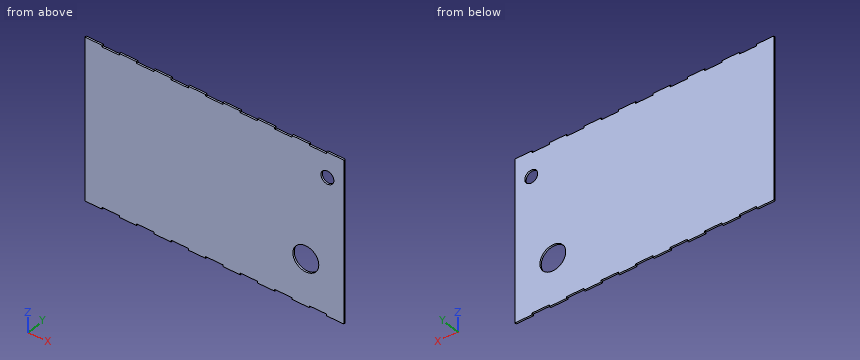
```python
from build123d import *

# Parameters (mm, degrees)
SKETCH1_W               = 300
SKETCH1_H               = 188
BOSS_EXTRUDE1_DEPTH     = 2
SKETCH2_W               = 20
SKETCH2_H               = 2
CUT_EXTRUDE1_DEPTH      = 4
LPATTERN1_COUNT         = 8
LPATTERN1_PITCH         = 40
MIRROR1_COPY_1_SKETCH_W = 20
MIRROR1_COPY_1_SKETCH_H = 2
MIRROR1_COPY_1_DEPTH    = 4
MIRROR1_COPY_2_SKETCH_W = 20
MIRROR1_COPY_2_SKETCH_H = 2
MIRROR1_COPY_2_DEPTH    = 4
MIRROR1_COPY_3_SKETCH_W = 20
MIRROR1_COPY_3_SKETCH_H = 2
MIRROR1_COPY_3_DEPTH    = 4
MIRROR1_COPY_4_SKETCH_W = 20
MIRROR1_COPY_4_SKETCH_H = 2
MIRROR1_COPY_4_DEPTH    = 4
MIRROR1_COPY_5_SKETCH_W = 20
MIRROR1_COPY_5_SKETCH_H = 2
MIRROR1_COPY_5_DEPTH    = 4
MIRROR1_COPY_6_SKETCH_W = 20
MIRROR1_COPY_6_SKETCH_H = 2
MIRROR1_COPY_6_DEPTH    = 4
MIRROR1_COPY_7_SKETCH_W = 20
MIRROR1_COPY_7_SKETCH_H = 2
MIRROR1_COPY_7_DEPTH    = 4
SKETCH4_R               = 7.5
SKETCH4_R_2             = 15
CUT_EXTRUDE2_DEPTH      = 3


with BuildPart() as part:
    # Sketch1 → Boss-Extrude1 (new body)
    with BuildSketch(Plane(origin=(0, 0, 0), x_dir=(1, 0, 0), z_dir=(0, 1, 0))):
        with Locations((-74.28137931, -28.264827586)):
            Rectangle(SKETCH1_W, SKETCH1_H)
    extrude(amount=BOSS_EXTRUDE1_DEPTH)

    # Sketch2 → Cut-Extrude1 (cut)
    with BuildSketch(Plane(origin=(0, 2, 0), x_dir=(1, 0, 0), z_dir=(0, 1, 0))):
        with Locations((-194.28137931, -121.264827586)):
            Rectangle(SKETCH2_W, SKETCH2_H)
    cut_extrude1 = extrude(amount=-CUT_EXTRUDE1_DEPTH, mode=Mode.SUBTRACT)

    # LPattern1: Cut-Extrude1 ×8
    with Locations(*[(i * LPATTERN1_PITCH, 0, 0) for i in range(1, LPATTERN1_COUNT)]):
        add(cut_extrude1, mode=Mode.SUBTRACT)

    # Mirror1: Cut-Extrude1 across plane
    add(cut_extrude1.mirror(Plane.XY.offset(28.264827586)), mode=Mode.SUBTRACT)

    # Mirror1 copy 1 sketch → Mirror1 copy 1 (cut)
    with BuildSketch(Plane(origin=(40, 2, 56.529655172), x_dir=(1, 0, 0), z_dir=(0, 1, 0))):
        with Locations((-194.28137931, 121.264827586)):
            Rectangle(MIRROR1_COPY_1_SKETCH_W, MIRROR1_COPY_1_SKETCH_H)
    extrude(amount=-MIRROR1_COPY_1_DEPTH, mode=Mode.SUBTRACT)

    # Mirror1 copy 2 sketch → Mirror1 copy 2 (cut)
    with BuildSketch(Plane(origin=(80, 2, 56.529655172), x_dir=(1, 0, 0), z_dir=(0, 1, 0))):
        with Locations((-194.28137931, 121.264827586)):
            Rectangle(MIRROR1_COPY_2_SKETCH_W, MIRROR1_COPY_2_SKETCH_H)
    extrude(amount=-MIRROR1_COPY_2_DEPTH, mode=Mode.SUBTRACT)

    # Mirror1 copy 3 sketch → Mirror1 copy 3 (cut)
    with BuildSketch(Plane(origin=(120, 2, 56.529655172), x_dir=(1, 0, 0), z_dir=(0, 1, 0))):
        with Locations((-194.28137931, 121.264827586)):
            Rectangle(MIRROR1_COPY_3_SKETCH_W, MIRROR1_COPY_3_SKETCH_H)
    extrude(amount=-MIRROR1_COPY_3_DEPTH, mode=Mode.SUBTRACT)

    # Mirror1 copy 4 sketch → Mirror1 copy 4 (cut)
    with BuildSketch(Plane(origin=(160, 2, 56.529655172), x_dir=(1, 0, 0), z_dir=(0, 1, 0))):
        with Locations((-194.28137931, 121.264827586)):
            Rectangle(MIRROR1_COPY_4_SKETCH_W, MIRROR1_COPY_4_SKETCH_H)
    extrude(amount=-MIRROR1_COPY_4_DEPTH, mode=Mode.SUBTRACT)

    # Mirror1 copy 5 sketch → Mirror1 copy 5 (cut)
    with BuildSketch(Plane(origin=(200, 2, 56.529655172), x_dir=(1, 0, 0), z_dir=(0, 1, 0))):
        with Locations((-194.28137931, 121.264827586)):
            Rectangle(MIRROR1_COPY_5_SKETCH_W, MIRROR1_COPY_5_SKETCH_H)
    extrude(amount=-MIRROR1_COPY_5_DEPTH, mode=Mode.SUBTRACT)

    # Mirror1 copy 6 sketch → Mirror1 copy 6 (cut)
    with BuildSketch(Plane(origin=(240, 2, 56.529655172), x_dir=(1, 0, 0), z_dir=(0, 1, 0))):
        with Locations((-194.28137931, 121.264827586)):
            Rectangle(MIRROR1_COPY_6_SKETCH_W, MIRROR1_COPY_6_SKETCH_H)
    extrude(amount=-MIRROR1_COPY_6_DEPTH, mode=Mode.SUBTRACT)

    # Mirror1 copy 7 sketch → Mirror1 copy 7 (cut)
    with BuildSketch(Plane(origin=(280, 2, 56.529655172), x_dir=(1, 0, 0), z_dir=(0, 1, 0))):
        with Locations((-194.28137931, 121.264827586)):
            Rectangle(MIRROR1_COPY_7_SKETCH_W, MIRROR1_COPY_7_SKETCH_H)
    extrude(amount=-MIRROR1_COPY_7_DEPTH, mode=Mode.SUBTRACT)

    # Sketch4 → Cut-Extrude2 (cut, through all)
    with BuildSketch(Plane.XZ):
        with Locations((56.71862069, 93.264827586)):
            Circle(SKETCH4_R)
        with Locations((31.71862069, -11.735172414)):
            Circle(SKETCH4_R_2)
    extrude(amount=-CUT_EXTRUDE2_DEPTH, mode=Mode.SUBTRACT)


solid = part.part
```
The model under review builds one solid part; all positions refer to its coordinate system, in mm. Round coordinates to 2 decimals unless told otherwise and drop trailing zeros. Loops run counter-clockwise (first coordinate to the right, second up) from the corner with the lowest first, then second, coordinate; pieces in that order, holes last. Notation, with made-up numbers: (78.5, -36) -> (98.5, -36) arc R23 ccw to (98.5, -2) -> close; hole circle Ø11 at (-7.75, 0.25). An arc over 180 degrees is marked (long way). Answer as a JSON object with one key per item and string values. Group by question number.
1) We need section B-B on x = -197. Write out the cut boundary in (y, z).
2) We need section C-C on y = 0.8. Give the number of separate pieces and of enclosed holes in the cut face, then the cut area to 3 significant figures.
3) For pin 1 Ø0.6 at (x, y) = (-76.5, 1) entering from -Z; pin 2 Ø0.6 at (x, y) = (-34, 1) entering from +Z, all flat-tipped, find the tip position at first contact; note any pin that passes through.
4) For line 1 (Z direction, x = -164, y = 1.5); line 2 (X direction, y = 1.4, z = 99); line 3 (X direction, y = 0.4, z = -4.5), list the stretches that pass through material, from the lowest coordinate up. Write a range as [from, to].
5) We need section A-A on x = 42.5. Write out the cut boundary in (y, z).
Result set:
{
 "1": {"outline": "(0, -63.74) -> (2, -63.74) -> (2, 120.26) -> (0, 120.26) -> close"},
 "2": {"separate pieces": "1", "enclosed holes": "2", "area": "55,000 mm²"},
 "3": {"pin 1": "z = -63.74", "pin 2": "z = 120.26"},
 "4": {"line 1": "[-63.74, 120.26]", "line 2": "[-224.28, 51.89], [61.55, 75.72]", "line 3": "[-224.28, 18.58], [44.86, 75.72]"},
 "5": {"outline": "(0, -63.74) -> (2, -63.74) -> (2, -22.16) -> (0, -22.16) -> close; (0, -1.31) -> (2, -1.31) -> (2, 120.26) -> (0, 120.26) -> close"}
}
